Model file for the job. Use its own axes, mm. Face numbers are marked on the shaded views. A direction names the side the tool comes from. Round coordinates to 2 decimals unless told otherwise and drop trailing zeros. Loops run counter-clockwise (first coordinate to the right, second up) from the corner with the lowest first, then second, coordinate; pieces in that order, holes last. Notation, with made-up numbers: M 2.5,24 L 22.5,24 A18 ccw 22.5,32 Z; hole C -28.5,86 d7. An arc over 180 degrees is marked long. Answer in a Markdown table with one row per item.
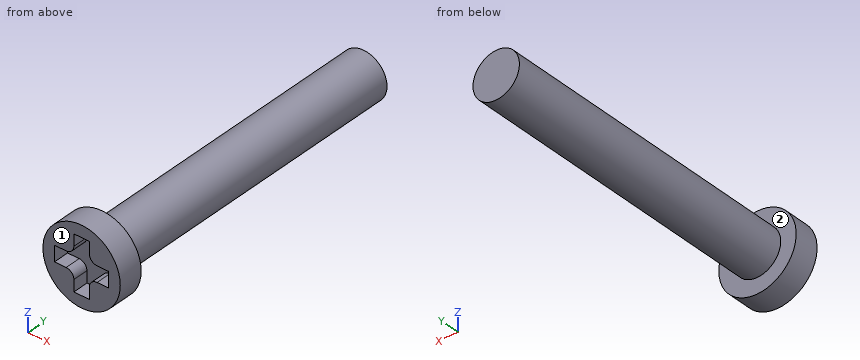
from build123d import *

# Parameters (mm, degrees)
SKETCH_1_R          = 2.5
EXTRUDE_1_DEPTH     = 1.6
SKETCH_2_R          = 1.5
EXTRUDE_2_DEPTH     = 20
CUT_EXTRUDE_1_DEPTH = 1


with BuildPart() as part:
    # 草图1 → 凸台-拉伸1 (new body)
    with BuildSketch(Plane(origin=(0, 0, 0), x_dir=(1, 0, 0), z_dir=(0, 1, 0))):
        Circle(SKETCH_1_R)
    extrude(amount=EXTRUDE_1_DEPTH)

    # 草图2 → 凸台-拉伸2 (add)
    with BuildSketch(Plane(origin=(0, 1.6, 0), x_dir=(1, 0, 0), z_dir=(0, 1, 0))):
        Circle(SKETCH_2_R)
    extrude(amount=EXTRUDE_2_DEPTH)

    # 草图3 → 切除-拉伸1 (cut)
    with BuildSketch(Plane.XZ):
        with BuildLine():
            Line((-0.5, 1), (-0.5, 1.75))
            Line((-0.5, 1.75), (0.5, 1.75))
            Line((0.5, 1.75), (0.5, 1))
            ThreePointArc((0.5, 1), (0.646446609, 0.646446609), (1, 0.5))
            Line((1, 0.5), (1.75, 0.5))
            Line((1.75, 0.5), (1.75, -0.5))
            Line((1.75, -0.5), (1, -0.5))
            ThreePointArc((1, -0.5), (0.646446609, -0.646446609), (0.5, -1))
            Line((0.5, -1), (0.5, -1.75))
            Line((0.5, -1.75), (-0.5, -1.75))
            Line((-0.5, -1.75), (-0.5, -1))
            ThreePointArc((-0.5, -1), (-0.646446609, -0.646446609), (-1, -0.5))
            Line((-1, -0.5), (-1.75, -0.5))
            Line((-1.75, -0.5), (-1.75, 0.5))
            Line((-1.75, 0.5), (-1, 0.5))
            ThreePointArc((-1, 0.5), (-0.646446609, 0.646446609), (-0.5, 1))
        make_face()
    extrude(amount=-CUT_EXTRUDE_1_DEPTH, mode=Mode.SUBTRACT)


solid = part.part
1. Saw through at B-B (z = 0). Write the cut outline in (x, y).
Verdict:
| item | result |
|---|---|
| outline | M -2.5,0 L -1.75,0 L -1.75,1 L 1.75,1 L 1.75,0 L 2.5,0 L 2.5,1.6 L 1.5,1.6 L 1.5,21.6 L -1.5,21.6 L -1.5,1.6 L -2.5,1.6 Z |
2. Saw through at A-A (x = 0). Write the cut outline in (y, z), and give its area (3 significant figures).
Verdict:
| item | result |
|---|---|
| outline | M 0,-2.5 L 1.6,-2.5 L 1.6,-1.5 L 21.6,-1.5 L 21.6,1.5 L 1.6,1.5 L 1.6,2.5 L 0,2.5 L 0,1.75 L 1,1.75 L 1,-1.75 L 0,-1.75 Z |
| area | 64.5 mm² |
3. Tool access for the marked faces 1 and 2: list every direction of +Z, -Z, +X, -X, +Y, -Y with a clear straight run to the whole face (end or side of a thin tool).
Verdict:
| item | result |
|---|---|
| face 1 | +Z, -Z, +X, -X, -Y |
| face 2 | +Y |
4. Wall check: probe 1 along Y at (x, z) = (-2.05, 0.4); probe 2 along Y at (x, z) = (1.2, 0); probe 3 along Z at (x, y) = (0.7, 9). Give the ranges that are in metal, low to high.
Verdict:
| item | result |
|---|---|
| probe 1 | y = 0 to 1.6 |
| probe 2 | y = 1 to 21.6 |
| probe 3 | z = -1.33 to 1.33 |
5. Saw through at C-C (y = 17.5). Write the cut outline in (x, z), and give its area (3 significant figures).
Verdict:
| item | result |
|---|---|
| outline | C 0,0 d3 |
| area | 7.07 mm² |
6. Pin check, flat tips, straight feed: pin 1 (1 mm diameter, centred on y = 9, z = 0.5, fed in from -X); pin 2 (1 mm diameter, centred on x = -1, y = 6.5, fed in from -Z); pin 3 (0.8 mm diameter, centred on x = 1.5, y = 0.5, fed in from -Z) (3 decimals). Stop position of each tip, or through.
Verdict:
| item | result |
|---|---|
| pin 1 | stops at x = -1.5 |
| pin 2 | stops at z = -1.41 |
| pin 3 | stops at z = -2.245 |
